Geometry: final body of the model. Coordinates: model frame, mm. A direction names the side the tool comes from. Coordinates: 2 decimals unless noted, no trailing zeros. Loops run counter-clockwise (first coordinate to the right, second up) from the corner with the lowest first, then second, coordinate; pieces in that order, holes last. Notation, with made-up numbers: M 30.5,32.25 L 71.5,32.25 A18 ccw 71.5,42.25 Z; hole C 68,17 d8. An arc over 180 degrees is marked long. Write item = value, one per line. Start each with the question number.
Autodesk Inventor part; units mm, degrees
ref_plane "YZ Plane" through (0, 0, 0) normal (1, 0, 0) x (0, 1, 0)
ref_plane "XZ Plane" through (0, 0, 0) normal (0, 1, 0) x (-1, 0, 0)
ref_plane "XY Plane" through (0, 0, 0) normal (0, 0, 1) x (1, 0, 0)
sketch "Эскиз1" plane through (0, 0, 0) normal (0, 0, 1) x (1, 0, 0)
  line L0 (-7, -3.5) -> (7, -3.5) construction
  line L1 (7, -3.5) -> (7, 3.5)
  line L2 (7, 3.5) -> (-7, 3.5)
  line L3 (-7, 3.5) -> (-7, -3.5)
  line L4 (-7, -3.5) -> (7, 3.5) construction
  line L5 (7, -3.5) -> (-7, 3.5) construction
  line L6 (0, -3.5) -> (0, -12.5) construction
  line L7 (-7, -3.5) -> (-3.289, -13.697)
  line L8 (7, -3.5) -> (3.289, -13.697)
  arc A0 (-3.289, -13.697) -> (3.289, -13.697) centre (0, -12.5) ccw
  point P0 (0, 0)
  point P1 (0, 0)
  point P2 (0, 0)
  point P3 (0, 0)
  dimension "d0" = 14
  dimension "d1" = 7
  dimension "d4" = 9
  dimension "d5" = 3.5
extrude "Выдавливание1" add sketch "Эскиз1" along normal blind 1.5
sketch "Эскиз4" plane through (0, 0, 1.5) normal (0, 0, 1) x (1, 0, 0)
  line L0 (7, 3.5) -> (-7, 3.5)
  line L1 (7, -3.5) -> (7, 3.5)
  line L2 (-7, 3.5) -> (-7, -3.5)
  line L3 (-7, -3.5) -> (7, -3.5)
  point P0 (0, 0)
extrude "Выдавливание6" add sketch "Эскиз4" along normal blind 3.2
sketch "Эскиз2" plane through (0, 0, 1.5) normal (0, 0, 1) x (1, 0, 0)
  arc A0 (-3.289, -13.697) -> (3.289, -13.697) centre (0, -12.5) ccw construction
  circle A1 centre (0, -12.5) radius 1.25
  point P0 (0, 0)
  dimension "d8" = 2.5
extrude "Выдавливание9" add sketch "Эскиз2" along normal blind 5
fillet "Сопряжение1" radius 3.5 2 edges at (7, 3.5, 2.35) (-7, 3.5, 2.35)
sketch "Эскиз5" plane through (0, 0, 4.7) normal (0, 0, 1) x (1, 0, 0)
  circle A0 centre (0, -9.5) radius 1.5 construction
  line L0 (7, -3.5) -> (-7, -3.5) construction
  line L1 (0, -3.5) -> (0, 3.5) construction
  line L2 (-7, 3.5) -> (7, 3.5) construction
  circle A1 centre (3.5, 0) radius 0.5
  line L3 (3.5, 3.5) -> (3.5, 0) construction
  line L4 (3.5, 0) -> (0, 0) construction
  circle A2 centre (-3.5, 0) radius 0.5
  dimension "d34" = 1
hole "Отверстие1" at (-3.5, 0, 4.7) at (3.5, 0, 4.7) direction (0, 0, -1) diameter 1 end through all countersink diameter 1.5 countersink angle 90
properties part number "переходник"
Item 1: Reachability of faces 1 (the flat face through (0, -4, 0)), 2 (the cylindrical face through (-0.16, -13.74, 3.96)), 3 (the flat face through (0, 0, 4.7)) from +Z, -Z, +X, -X, +Y, -Y: full face, straight path, thin tool, end or side. Return the list, or none.
Item 2: Line query: line 1 (X direction, y = 0, z = 3.2); line 2 (Y direction, x = -3.5, z = 2.35); line 3 (Y direction, x = 0, z = 3.25). Output: solid intervals per line, ascending. Write a range as from..to.
Item 3: Section query D-D (y = -12.5). Return the cut outline in (x, z), plus the area to 3 significant figures.
Item 4: First-contact query: pin 1 (1.5 mm diameter, centred on y = -12.5, z = 5.5, fed in from +X); pin 2 (2.5 mm diameter, centred on x = 1.5, z = 3, fed in from -Y); pin 3 (5 mm diameter, centred on x = 4, y = -8, fed in from +Z). Flat tips, straight axial feed; report the tip coordinate or a pass-through.
Item 5: Section query C-C (z = 5.5). Return the cut outline in (x, y).
Item 6: Section query B-B (x = 0). Return the cut outline in (y, z).
Item 7: Section query A-A (z = 2). Return the cut outline in (x, y), plus the area to 3 significant figures.
Item 8: Pull-direction query (X, two-part tool) for faces 4 (the cylindrical face through (3, 0, 2)), 5 (the cylindrical face through (0, -16, 1)), 6 (the cylindrical face through (-4, 0, 2)), 7 (the flat face through (0, -3.5, 3)); classes: released by +X, released by -X, zero draft, split by the parting line, or undercut.
Verdict:
q1.face_1 = -Z, +X, -X, +Y, -Y
q1.face_2 = +Z
q1.face_3 = +Z, +X, -X, +Y
q2.line_1 = -7..-4, -3..3, 4..7
q2.line_2 = -3.5..-0.5, 0.5..3.5
q2.line_3 = -13.75..-11.25, -3.5..3.5
q3.outline = M -3.72,0 L 3.72,0 L 3.72,1.5 L 1.25,1.5 L 1.25,6.5 L -1.25,6.5 L -1.25,1.5 L -3.72,1.5 Z
q3.area = 23.7 mm2
q4.pin_1 = 1.25
q4.pin_2 = -13.72
q4.pin_3 = 1.5
q5.outline = C 0,-12.5 d2.5
q6.outline = M -16,0 L 3.5,0 L 3.5,4.7 L -3.5,4.7 L -3.5,1.5 L -11.25,1.5 L -11.25,6.5 L -13.75,6.5 L -13.75,1.5 L -16,1.5 Z
q7.outline = M -7,-3.5 L 7,-3.5 L 7,0 A3.5 ccw 3.5,3.5 L -3.5,3.5 A3.5 ccw -7,0 Z; C 0,-12.5 d2.5; hole C -3.5,0 d1; hole C 3.5,0 d1
q7.area = 96.1 mm2
q8.face_4 = undercut
q8.face_5 = split by the parting line
q8.face_6 = undercut
q8.face_7 = zero draft
